Part model, mm, in its own coordinate system. A direction names the side the tool comes from. Round coordinates to 2 decimals unless told otherwise and drop trailing zeros. Loops run counter-clockwise (first coordinate to the right, second up) from the corner with the lowest first, then second, coordinate; pieces in that order, holes last. Notation, with made-up numbers: M 64,36 L 112,36 A18 cw 112,55 Z; hole C -29,19 d8. An arc over 180 degrees is marked long. Answer as CSV lines item,"result". Start each with the question number.
Item 1: Band-saw the part on C-C (y = 61). Give the cut face in (x, z) (3 decimals).
Item 2: Drop flat-ended pins along their axis: pin 1 Ø10 at (x, y) = (56, -57.5) entering from +Z; pin 2 Ø8 at (x, y) = (-28, 43.5) entering from -Z; pin 3 Ø11 at (x, z) = (-94.5, 28) entering from +Y; pin 4 Ø10 at (x, z) = (-75, 46) entering from +Y. Give the stop position or say it passes through.
Item 3: Mould opens along Z. For faces 4 (the flat face through (101.6, -31, 3)), 5 (the flat face through (-84.836, -81, 21)), 6 (the flat face through (92, -99, 56.642)) say: pulls with the +Z half, pulls with the -Z half, needs draft (parallel to the pull), parting line crosses it, or undercut.
Item 4: Band-saw the part on A-A (z = 34.5). Give the cut face in (x, y), and give its area (3 significant figures).
Item 5: Band-saw the part on D-D (y = -27.5). Give the cut face in (x, z) (3 decimals), and give its area (3 significant figures).
Item 6: Band-saw the part on B-B (x = -20.5). Give the cut face in (y, z).
Item 7: Wall check: line 1 (X direction, y = -75.5, z = 21); line 2 (X direction, y = -99.3, z = 40.84); line 3 (Z direction, x = -76.5, y = -86). Give the ranges that are in metal, low to high.
Item 8: Which spindle directions (+Z, -Z, +X, -X, +Y, -Y) get a long thin tool onto all of the face, cutting with end or side? Do faces 1 (the flat face through (34.5, 47.2, 2.5)), 2 (the flat face through (-84.836, -84, 49)), 3 (the flat face through (85.165, -76.104, 30.5)). Say none if no direction does.
```python
from build123d import *

# Parameters (mm, degrees)
SKETCH1_W           = 203.2
SKETCH1_H           = 203.2
SKETCH1_R           = 1.5
BOSS_EXTRUDE1_DEPTH = 5.08
SKETCH2_W           = 13.97
SKETCH2_H           = 5.08
BOSS_EXTRUDE2_DEPTH = 51.562
CUT_EXTRUDE1_REACH  = 231.744
SKETCH3_R           = 2.159
CUT_EXTRUDE4_DEPTH  = 3
BOSS_EXTRUDE3_REACH = 181.07
SKETCH12_W          = 3.81
SKETCH12_H          = 31.496
SKETCH14_W          = 15.49
SKETCH14_H          = 36.576
CUT_EXTRUDE5_DEPTH  = 53.086
SKETCH15_R          = 1.6
CUT_EXTRUDE6_DEPTH  = 10
CUT_EXTRUDE7_DEPTH  = 2.3
BOSS_EXTRUDE5_START = -13.97
SKETCH17_W          = 51.562
SKETCH17_H          = 5.08
BOSS_EXTRUDE5_DEPTH = 5


with BuildPart() as part:
    # Sketch1 → Boss-Extrude1 (new body)
    with BuildSketch(Plane.XY):
        Rectangle(SKETCH1_W, SKETCH1_H)
        Polygon((-82.55, -68.309231637), (-82.55, -9.525), (-23.765768363, -9.525), align=None, mode=Mode.SUBTRACT)
        Polygon((-51.657605136, -65.024), (-9.525, -22.891394864), (-9.525, -65.024), align=None, mode=Mode.SUBTRACT)
        Polygon((9.525, -82.55), (9.525, -22.225), (69.85, -82.55), align=None, mode=Mode.SUBTRACT)
        Polygon((82.55, -68.309231637), (65.605706321, -51.364937958), (65.605706321, -9.525), (82.55, -9.525), align=None, mode=Mode.SUBTRACT)
        Polygon((58.758115986, -44.517347622), (23.765768363, -9.525), (58.758115986, -9.525), align=None, mode=Mode.SUBTRACT)
        Polygon((-23.765768363, 9.525), (-82.55, 9.525), (-82.55, 68.309231637), align=None, mode=Mode.SUBTRACT)
        Polygon((-9.525, 22.225), (-69.85, 82.55), (-9.525, 82.55), align=None, mode=Mode.SUBTRACT)
        with Locations((-63.5, 97.79)):
            Circle(SKETCH1_R, mode=Mode.SUBTRACT)
        with Locations((0, 25.4)):
            Circle(SKETCH1_R, mode=Mode.SUBTRACT)
        Polygon((58.758115986, 44.517347622), (58.758115986, 9.525), (23.765768363, 9.525), align=None, mode=Mode.SUBTRACT)
        Polygon((9.525, 82.55), (58.758115986, 82.55), (58.758115986, 71.458115986), (9.525, 22.225), align=None, mode=Mode.SUBTRACT)
        Polygon((82.55, 9.525), (65.605706321, 9.525), (65.605706321, 51.364937958), (82.55, 68.309231637), align=None, mode=Mode.SUBTRACT)
        with Locations((0, 76.2)):
            Circle(SKETCH1_R, mode=Mode.SUBTRACT)
        Polygon((65.605706321, 78.305706321), (65.605706321, 82.55), (69.85, 82.55), align=None, mode=Mode.SUBTRACT)
        with Locations((63.5, 97.79)):
            Circle(SKETCH1_R, mode=Mode.SUBTRACT)
    extrude(amount=BOSS_EXTRUDE1_DEPTH)

    # Sketch2 → Boss-Extrude2 (add)
    with BuildSketch(Plane.XY.offset(5.08)):
        Polygon((-101.6, -96.52), (-101.6, -101.6), (-31.75, -101.6), (-31.75, -65.024), (-34.544, -65.024), (-34.544, -96.409365186), (-84.836, -96.409365186), (-84.836, -65.024), (-87.63, -65.024), (-87.63, -96.52), align=None)
        with Locations((94.615, -99.06)):
            Rectangle(SKETCH2_W, SKETCH2_H)
    extrude(amount=BOSS_EXTRUDE2_DEPTH)

    # Sketch3 → Cut-Extrude1 (cut, up to next)
    with BuildSketch(Plane(origin=(0, -96.52, 0), x_dir=(1, 0, 0), z_dir=(0, 1, 0)), mode=Mode.PRIVATE) as cut_extrude1_sk1:
        with Locations(Location((-94.615, -11.43, 0), (0, 0, 270))):
            Circle(SKETCH3_R)
    cut_extrude1_tool1 = extrude(cut_extrude1_sk1.sketch, amount=-CUT_EXTRUDE1_REACH, mode=Mode.PRIVATE) & part.part
    # Sketch3 → Cut-Extrude1 (cut, up to next)
    with BuildSketch(Plane(origin=(0, -96.52, 0), x_dir=(1, 0, 0), z_dir=(0, 1, 0)), mode=Mode.PRIVATE) as cut_extrude1_sk2:
        with Locations(Location((94.615, -11.43, 0), (0, 0, 270))):
            Circle(SKETCH3_R)
    cut_extrude1_tool2 = extrude(cut_extrude1_sk2.sketch, amount=-CUT_EXTRUDE1_REACH, mode=Mode.PRIVATE) & part.part
    # Sketch3 → Cut-Extrude1 (cut, up to next)
    with BuildSketch(Plane(origin=(0, -96.52, 0), x_dir=(1, 0, 0), z_dir=(0, 1, 0)), mode=Mode.PRIVATE) as cut_extrude1_sk3:
        with Locations(Location((94.615, -40.84, 0), (0, 0, 270))):
            Circle(SKETCH3_R)
    cut_extrude1_tool3 = extrude(cut_extrude1_sk3.sketch, amount=-CUT_EXTRUDE1_REACH, mode=Mode.PRIVATE) & part.part
    # Sketch3 → Cut-Extrude1 (cut, up to next)
    with BuildSketch(Plane(origin=(0, -96.52, 0), x_dir=(1, 0, 0), z_dir=(0, 1, 0)), mode=Mode.PRIVATE) as cut_extrude1_sk4:
        with Locations(Location((-94.615, -40.84, 0), (0, 0, 270))):
            Circle(SKETCH3_R)
    cut_extrude1_tool4 = extrude(cut_extrude1_sk4.sketch, amount=-CUT_EXTRUDE1_REACH, mode=Mode.PRIVATE) & part.part
    add(cut_extrude1_tool1.solids().sort_by_distance((-94.615, -96.52, 11.43))[0], mode=Mode.SUBTRACT)
    add(cut_extrude1_tool2.solids().sort_by_distance((94.615, -96.52, 11.43))[0], mode=Mode.SUBTRACT)
    add(cut_extrude1_tool3.solids().sort_by_distance((94.615, -96.52, 40.84))[0], mode=Mode.SUBTRACT)
    add(cut_extrude1_tool4.solids().sort_by_distance((-94.615, -96.52, 40.84))[0], mode=Mode.SUBTRACT)

    # Sketch11 → Cut-Extrude4 (cut)
    with BuildSketch(Plane.XY.offset(5.08)):
        Polygon((-61.86898549, 94.965), (-60.237970979, 97.79), (-61.86898549, 100.615), (-65.13101451, 100.615), (-66.762029021, 97.79), (-65.13101451, 94.965), align=None)
        Polygon((65.13101451, 94.965), (61.86898549, 94.965), (60.237970979, 97.79), (61.86898549, 100.615), (65.13101451, 100.615), (66.762029021, 97.79), align=None)
    extrude(amount=-CUT_EXTRUDE4_DEPTH, mode=Mode.SUBTRACT)

    # Sketch12 → Boss-Extrude3 (add, up to next)
    with BuildSketch(Plane.ZY.offset(34.544), mode=Mode.PRIVATE) as boss_extrude3_sk1:
        with Locations((39.243, -80.772)):
            Rectangle(SKETCH12_W, SKETCH12_H)
    boss_extrude3_tool1 = extrude(boss_extrude3_sk1.sketch, amount=BOSS_EXTRUDE3_REACH, mode=Mode.PRIVATE) - part.part
    add(boss_extrude3_tool1.solids().sort_by_distance((-34.544, -80.772, 39.243))[0])

    # Sketch14 → Cut-Extrude5 (cut)
    with BuildSketch(Plane(origin=(-31.75, 0, 0), x_dir=(0, 0, -1), z_dir=(1, 0, 0))):
        with Locations((-48.897, -83.312)):
            Rectangle(SKETCH14_W, SKETCH14_H)
    extrude(amount=-CUT_EXTRUDE5_DEPTH, mode=Mode.SUBTRACT)

    # Sketch15 → Cut-Extrude6 (cut)
    with BuildSketch(Plane.XY.offset(5.08)):
        with Locations((61.285165756, 2.786448521)):
            Circle(SKETCH15_R)
        with Locations((80.785165756, 2.786448521)):
            Circle(SKETCH15_R)
        with Locations((80.785165756, -38.937697653)):
            Circle(SKETCH15_R)
        with Locations((61.285165756, -38.937697653)):
            Circle(SKETCH15_R)
    extrude(amount=-CUT_EXTRUDE6_DEPTH, mode=Mode.SUBTRACT)

    # Sketch16 → Cut-Extrude7 (cut)
    with BuildSketch(Plane(origin=(0, 0, 0), x_dir=(-1, 0, 0), z_dir=(0, 0, -1))):
        Polygon((-1.58771324, 73.45), (1.58771324, 73.45), (3.175426481, 76.2), (1.58771324, 78.95), (-1.58771324, 78.95), (-3.175426481, 76.2), align=None)
        Polygon((-3.175426481, 25.4), (-1.58771324, 22.65), (1.58771324, 22.65), (3.175426481, 25.4), (1.58771324, 28.15), (-1.58771324, 28.15), align=None)
        Polygon((-64.460592236, 2.786448521), (-62.872878996, 0.036448521), (-59.697452515, 0.036448521), (-58.109739275, 2.786448521), (-59.697452515, 5.536448521), (-62.872878996, 5.536448521), align=None)
        Polygon((-83.960592236, 2.786448521), (-82.372878996, 0.036448521), (-79.197452515, 0.036448521), (-77.609739275, 2.786448521), (-79.197452515, 5.536448521), (-82.372878996, 5.536448521), align=None)
        Polygon((-64.460592236, -38.937697653), (-62.872878996, -41.687697653), (-59.697452515, -41.687697653), (-58.109739275, -38.937697653), (-59.697452515, -36.187697653), (-62.872878996, -36.187697653), align=None)
    extrude(amount=-CUT_EXTRUDE7_DEPTH, mode=Mode.SUBTRACT)

    # Sketch17 → Boss-Extrude5 (add)
    with BuildSketch(Plane(origin=(101.6, 0, 0), x_dir=(0, 0, -1), z_dir=(1, 0, 0)).offset(BOSS_EXTRUDE5_START)):
        Polygon((-5.08, -56.252401603), (-56.642, -96.52), (-5.08, -96.52), align=None)
        with Locations((-30.861, -99.06)):
            Rectangle(SKETCH17_W, SKETCH17_H)
    extrude(amount=-BOSS_EXTRUDE5_DEPTH)


solid = part.part
```
Answer block:
1,outline,"M -101.6,0 L -82.55,0 L -82.55,5.08 L -101.6,5.08 Z; M -75.241,0 L -48.3,0 L -48.3,5.08 L -75.241,5.08 Z; M -9.525,0 L 9.525,0 L 9.525,5.08 L -9.525,5.08 Z; M 48.3,0 L 75.241,0 L 75.241,5.08 L 48.3,5.08 Z; M 82.55,0 L 101.6,0 L 101.6,5.08 L 82.55,5.08 Z"
2,pin 1,"stops at z = 5.08"
2,pin 2,"stops at z = 0"
2,pin 3,"stops at y = -96.52"
2,pin 4,"stops at y = -65.02"
3,face 4,"needs draft"
3,face 5,"undercut"
3,face 6,"pulls with the +Z half"
4,outline,"M -101.6,-101.6 L -31.75,-101.6 L -31.75,-65.02 L -34.54,-65.02 L -34.54,-96.41 L -84.84,-96.41 L -84.84,-65.02 L -87.63,-65.02 L -87.63,-96.52 L -101.6,-96.52 Z; M 82.63,-101.6 L 101.6,-101.6 L 101.6,-96.52 L 87.63,-96.52 L 87.63,-79.23 L 82.63,-79.23 Z"
4,area,"719 mm^2"
5,outline,"M -101.6,0 L -82.55,0 L -82.55,5.08 L -101.6,5.08 Z; M -41.741,0 L -14.134,0 L -14.134,5.08 L -41.741,5.08 Z; M -9.525,0 L 9.525,0 L 9.525,5.08 L -9.525,5.08 Z; M 14.8,0 L 41.741,0 L 41.741,5.08 L 14.8,5.08 Z; M 58.758,0 L 65.606,0 L 65.606,5.08 L 58.758,5.08 Z; M 82.55,0 L 101.6,0 L 101.6,5.08 L 82.55,5.08 Z"
5,area,"602 mm^2"
6,outline,"M -101.6,0 L -65.02,0 L -65.02,5.08 L -101.6,5.08 Z; M -33.87,0 L 33.2,0 L 33.2,5.08 L -33.87,5.08 Z; M 82.55,0 L 101.6,0 L 101.6,5.08 L 82.55,5.08 Z"
7,line 1,"x = -87.63 to -84.84, -34.54 to -31.75, 82.63 to 87.63"
7,line 2,"x = -101.6 to -96.77, -92.46 to -31.75, 82.63 to 92.46, 96.77 to 101.6"
7,line 3,"z = 0 to 5.08, 37.34 to 41.15"
8,face 1,"+Z, -Z"
8,face 2,"+Z, +Y, -Y"
8,face 3,"+Z, +X, +Y"
